from build123d import *

# Parameters (mm, degrees)
F1_DEPTH   = 38.1
F2_R       = 9.525
F3_DEPTH   = 101.6
F1_FACE2_W = 38.1
F1_FACE2_H = 19.05
F5_DEPTH   = 152.4
F7_DEPTH   = 63.5
F9_DEPTH   = 50.8
F10_R      = 0.635
F11_DEPTH  = 1.6002


with BuildPart() as f1:
    # F0 (on Front) → F1 (new body)
    with BuildSketch(Plane.XZ):
        Polygon((0, 63.5), (0, 0), (304.8, 0), (304.8, 19.05), align=None)
    extrude(amount=F1_DEPTH)

    # F2 (on face) → F3 (cut)
    with BuildSketch(Plane(origin=(0, 0, 0), x_dir=(0, -1, 0), z_dir=(-1, 0, 0))):
        with Locations((19.05, 38.1)):
            Circle(F2_R)
    extrude(amount=-F3_DEPTH, mode=Mode.SUBTRACT)

    # F4 (on face) + F1_face2 (on face) → F5 (cut)
    with BuildSketch(Plane(origin=(9.0675733107, 0, 62.1776455589), x_dir=(0.9895329811, 0, -0.1443068931), z_dir=(0.1443068931, 0, 0.9895329811))):
        Polygon((197.2606063151, -6.35), (197.2606063151, 0), (-9.1634877101, 0), (70.2606063151, -6.35), (95.6606063151, -6.35), align=None)
        Polygon((-9.1634877101, -38.1), (197.2606063151, -38.1), (197.2606063151, -31.75), (95.6606063151, -31.75), (70.2606063151, -31.75), align=None)
        Polygon((298.8606063151, -19.05), (298.8606063151, 0), (197.2606063151, 0), align=None)
        Polygon((298.8606063151, -38.1), (298.8606063151, -19.05), (197.2606063151, -38.1), align=None)
    with BuildSketch(Plane(origin=(304.8, -19.05, 9.525), x_dir=(0, 1, 0), z_dir=(1, 0, 0))):
        Rectangle(F1_FACE2_W, F1_FACE2_H)
    extrude(amount=-F5_DEPTH, dir=(0.1443068931, 0, 0.9895329811), mode=Mode.SUBTRACT)

    # F6 (on face) → F7 (cut)
    with BuildSketch(Plane(origin=(2.9374947207, -37.1300355722, -0.4283846468), x_dir=(0.9968855377, 0.0788568126, 0.0009098038), z_dir=(0.0788620609, -0.9968191957, -0.0115007172))):
        with BuildLine():
            ThreePointArc((34.5711449956, 8.0186913962), (31.3191065774, 9.3657298144), (32.6661449956, 6.1136913962))
            ThreePointArc((32.6661449956, 6.1136913962), (34.0131834138, 6.6716529781), (34.5711449956, 8.0186913962))
        make_face()
    extrude(amount=-F7_DEPTH, mode=Mode.SUBTRACT)

    # F8 (on face) → F9 (cut)
    with BuildSketch(Plane(origin=(13.4581916909, -72.5362607665, -1.9626529549), x_dir=(0.9832319067, 0.1822928664, 0.004932397), z_dir=(0.1823595835, -0.9828721869, -0.0265941059))):
        with BuildLine():
            ThreePointArc((241.2876717144, 3.947847759), (242.6407823243, 4.5024670011), (243.2020712552, 5.8528245695))
            ThreePointArc((243.2020712552, 5.8528245695), (239.953360186, 7.2031821379), (241.2876717144, 3.947847759))
        make_face()
    extrude(amount=-F9_DEPTH, mode=Mode.SUBTRACT)

    # F10 (on face) → F11 (cut)
    with BuildSketch(Plane(origin=(0, 0, 0), x_dir=(1, 0, 0), z_dir=(0, 0, -1))):
        with Locations((250.615478633, 18.1772389299)):
            Circle(F10_R)
    extrude(amount=-F11_DEPTH, mode=Mode.SUBTRACT)


solid = f1.part
The model under review builds one solid part; all positions refer to its coordinate system, in mm. A direction names the side the tool comes from. Give positions to 0.01 mm unless a question says otherwise; leave off trailing zeros. Write each loop counter-clockwise with the first axis right and the second up, starting at its lowest first coordinate (ties: lowest second). Pieces come first, ordered by that corner, then holes.
1. Add section C-C, the plane x = 233.5. Write out the cut boundary in (y, z), plus the area to 3 significant figures.
2. Add section D-D, the plane z = 38.1. Write out the cut boundary in (x, y) (3 decimals), plus the area to 3 significant figures.
3. Add section B-B, the plane z = 22. Write out the cut boundary in (x, y).
4. Add section A-A, the plane x = 64. Write out the cut boundary in (y, z) (3 decimals), plus the area to 3 significant figures.
5. Wall thickness on L1, parallel to Z at x = 94.5, y = -21; L2, parallel to Z at x = 48.5, y = -19.05 (3 decimals); L3, parallel to Z at x = 246.5, y = -27.5: over which ranges is each line inside the solid? List them lowest first.
6. For P1, Ø5, axis at x = 145, z = 44, coming from the -Y side; P2, Ø2, axis at x = 49.5, y = -10.5, coming from the -Z side; P3, Ø1.1, axis at x = 250.62, y = -18.18, coming from the -Z side; P4, Ø8, axis at x = 77, z = 39.5, coming from the +Y side, all flat-tipped, find the tip position at first contact; note any pin that passes through.
7. Tool access review of faces 1 (the cylindrical face through (50.089, -17.81, 47.544)), 2 (the flat face through (120.667, -18.783, 45.903)), 3 (the flat face through (0, -19, 25)), 4 (the flat face through (201.84, -34.97, 17.09)), 5 (the flat face through (201.84, -3.22, 17.09)): name each direction out of +Z, -Z, +X, -X, +Y, -Y from which nothing blocks a thin tool from reaching the whole face with its end or side.
8. Draft analysis for pull direction X (two halves, no side actions). For faces 6 (the flat face through (139, -31.75, 23)), 7 (the flat face through (138, -6.35, 23)), 8 (the flat face through (115, -19, 0)), 9 (the flat face through (101.6, -19, 38)), state which applies: +X half, -X half, draft (parallel to the pull), parting line (faces both ways), or undercut.
Worked answers:
1. outline: (-32.56, 29.45) - (-31.76, 0) - (-6.34, 0) - (-5.54, 29.45) - close
1. area: 772 mm2
2. outline: (0, -37.807) - (76.56, -31.75) - (174.171, -31.75) - (174.171, -6.35) - (76.56, -6.35) - (0, -0.293) - (0, -9.525) - (101.6, -9.525) - (101.6, -28.575) - (0, -28.575) - close
2. area: 2,950 mm2
3. outline: (0, -37.62) - (74.21, -31.75) - (202.56, -31.75) - (202.56, -38.1) - (284.57, -22.88) - (284.57, -15.22) - (202.56, 0) - (202.56, -6.35) - (74.21, -6.35) - (0, -0.48) - close
4. outline: (-32.929, 54.167) - (-32.304, 0) - (-5.796, 0) - (-5.171, 54.167) - close; hole circle Ø19.05 at (-19.05, 38.1)
4. area: 1,180 mm2
5. L1: z = 0 to 28.78, 47.42 to 49.72
5. L2: z = 0 to 28.575, 47.625 to 56.427
5. L3: z = 0 to 27.55
6. P1: stops at y = -31.75
6. P2: stops at z = 0
6. P3: stops at z = 1.6
6. P4: stops at y = -6.05
7. face 1: -X
7. face 2: +Z, +X, +Y, -Y
7. face 3: +Z, -Z, -X, +Y, -Y
7. face 4: +Z, -Y
7. face 5: +Z, +Y
8. face 6: undercut
8. face 7: undercut
8. face 8: draft
8. face 9: -X half
